```python
from build123d import *

# Parameters (mm, degrees)
SWEEP1_PROFILE_R = 1.65


with BuildPart() as part:
    # Sweep1: sweep along a path in Sketch1
    with BuildLine(Plane.XY) as sweep1_path:
        Line((4.249998297, 82.00000012), (4.249998297, 18.00000012))
        ThreePointArc((4.249998297, 18.00000012), (8.277280056, 8.277281879), (17.999998297, 4.25000012))
        Line((17.999998297, 4.25000012), (81.999998297, 4.25000012))
        ThreePointArc((81.999998297, 4.25000012), (91.722716538, 8.277281879), (95.749998297, 18.00000012))
        Line((95.749998297, 18.00000012), (95.749998297, 82.00000012))
        ThreePointArc((95.749998297, 82.00000012), (91.722716538, 91.722718361), (81.999998297, 95.75000012))
        Line((81.999998297, 95.75000012), (17.999998297, 95.75000012))
        ThreePointArc((17.999998297, 95.75000012), (8.277280056, 91.722718361), (4.249998297, 82.00000012))
    # Sweep1 profile (on start of the path) → Sweep1 (sweep)
    with BuildSketch(Plane(origin=(4.249998297, 82.00000012, 0), x_dir=(-1, 0, 0), z_dir=(0, -1, 0))):
        Circle(SWEEP1_PROFILE_R)
    sweep(path=sweep1_path.line)


solid = part.part
```
Work out the finished part from the listing and answer in its coordinate system (mm). Round coordinates to 2 decimals unless told otherwise and drop trailing zeros. Order: outer loops, then holes, each group sorted by start corner. A loop starts at its lowest first (then second) coordinate and runs counter-clockwise, first axis right, second up.
Q1. Find the intervals of material crossed by line 1 along X through (y, z) = (53, 0.2); line 2 along Y through (x, z) = (30.5, 0.1); line 3 along Y through (x, z) = (7.5, 0.35), in increasing order.
Solution:
line 1: x = 2.61 to 5.89, 94.11 to 97.39
line 2: y = 2.6 to 5.9, 94.1 to 97.4
line 3: y = 6.79 to 11.91, 88.09 to 93.21
Q2. Given pin 1 Ø1.5 at (y, z) = (73.5, 1.5) entering from +X, flat-ended and moving along its own axis, determine where the tip first touches the part or whether it passes through.
Solution:
pin 1: stops at x = 97.22
Q3. A cutting plane is placed at A-A, the plane z = 0. Determine the outline of the cut face in (x, y).
Solution:
outline: (2.6, 18) arc R15.4 ccw to (18, 2.6) - (82, 2.6) arc R15.4 ccw to (97.4, 18) - (97.4, 82) arc R15.4 ccw to (82, 97.4) - (18, 97.4) arc R15.4 ccw to (2.6, 82) - close; hole (5.9, 18) arc R12.1 ccw to (18, 5.9) - (82, 5.9) arc R12.1 ccw to (94.1, 18) - (94.1, 82) arc R12.1 ccw to (82, 94.1) - (18, 94.1) arc R12.1 ccw to (5.9, 82) - close
Q4. A cutting plane is placed at B-B, the plane y = 36. Determine the outline of the cut face in (x, z).
Solution:
outline: circle Ø3.3 at (4.25, 0); circle Ø3.3 at (95.75, 0)
Q5. The mould has two halves that part along X. Classify faces 1 (the cylindrical face through (50.448, 2.676, -0.496)), 2 (the cylindrical face through (5.9, 49.55, -0.07)): pulls with the +X half, pulls with the -X half, needs draft (parallel to the pull), parting line crosses it, or undercut.
Solution:
face 1: undercut
face 2: undercut
